The model under review builds one solid part; all positions refer to its coordinate system, in mm. A direction names the side the tool comes from. Round coordinates to 2 decimals unless told otherwise and drop trailing zeros. Write each loop counter-clockwise with the first axis right and the second up, starting at its lowest first coordinate (ties: lowest second). Pieces come first, ordered by that corner, then holes. Notation, with made-up numbers: (72.5, 55.5) -> (101.5, 55.5) arc R16 cw to (101.5, 74.5) -> close; hole circle Ø11 at (27, 71). An arc over 180 degrees is marked (long way). Answer as a JSON object with one key per item and string values. Group by question number.
1) Mouldability with a two-part tool opening along Y and no side actions: class faces 1 (the cylindrical face through (-3.955, 12.325, -5.158)), 2 (the flat face through (-8, 120, 0)), 3 (the flat face through (-8, 23, 0)), 4 (the cylindrical face through (-10.74, 59.51, -2.38)) as pulls with the +Y half, pulls with the -Y half, needs draft (parallel to the pull), parting line crosses it, or undercut.
2) We need section A-A, the plane x = 0. Write out the cut boundary in (y, z), then the cut area to 3 significant figures.
3) We need section D-D, the plane y = 69.5. Write out the cut boundary in (x, z).
4) We need section B-B, the plane z = 3.75. Write out the cut boundary in (x, y).
5) Insertion check: pin 1 Ø1.5 at (x, y) = (-6.5, 105.5) entering from -Z; pin 2 Ø6 at (x, z) = (0, 0.5) entering from +Y; pin 3 Ø10 at (y, z) = (40, -6.5) entering from +X; pin 4 Ø6 at (y, z) = (94.5, 5) entering from -X. Each pin has a flat end and moves straight along its axis. Give the tip position at first contact, or say it passes through.
6) We need section C-C, the plane y = 112. Write out the cut boundary in (x, z), then the cut area to 3 significant figures.
7) Machinability: for faces 5 (the cylindrical face through (0.33, 11.339, -7.493)), 6 (the flat face through (3, 0, -6)), 7 (the flat face through (3, 97, 8.2)), 8 (the flat face through (-5, 25, 5)), which of the approach directions +Z, -Z, +X, -X, +Y, -Y give a long, thin tool a straight path to every point of the face, cutting with its end or side? Answer none if there is none.
8) To check wall thickness, follow probe 1 along Y at (x, z) = (5.75, -9); probe 2 along X at (y, z) = (10.25, 0); probe 3 along X at (y, z) = (111, 0). State the ranges of each line that lie inside material, in increasing order. Write a range as [from, to].
from build123d import *

# Parameters (mm, degrees)
SKETCH1_R           = 7.5
SKETCH1_R_2         = 6.5
BOSS_EXTRUDE1_DEPTH = 23
SKETCH2_R           = 12.5
SKETCH2_R_2         = 6.5
BOSS_EXTRUDE2_DEPTH = 2
SKETCH3_R           = 12.5
SKETCH3_R_2         = 11
BOSS_EXTRUDE3_DEPTH = 70
SKETCH4_R           = 12.5
SKETCH4_R_2         = 7.5
BOSS_EXTRUDE4_DEPTH = 2
SKETCH5_R           = 8.5
SKETCH5_R_2         = 7.5
BOSS_EXTRUDE5_DEPTH = 23


with BuildPart() as part:
    # Sketch1 → Boss-Extrude1 (new body)
    with BuildSketch(Plane(origin=(0, 0, 0), x_dir=(1, 0, 0), z_dir=(0, 1, 0))):
        with Locations(Location((0, 0, 0), (0, 0, 270))):
            Circle(SKETCH1_R)
        with Locations(Location((0, 0, 0), (0, 0, 270))):
            Circle(SKETCH1_R_2, mode=Mode.SUBTRACT)
    extrude(amount=BOSS_EXTRUDE1_DEPTH)

    # Sketch2 → Boss-Extrude2 (add)
    with BuildSketch(Plane(origin=(0, 23, 0), x_dir=(1, 0, 0), z_dir=(0, 1, 0))):
        with Locations(Location((0, 0, 0), (0, 0, 270))):
            Circle(SKETCH2_R)
        with Locations(Location((0, 0, 0), (0, 0, 270))):
            Circle(SKETCH2_R_2, mode=Mode.SUBTRACT)
    extrude(amount=BOSS_EXTRUDE2_DEPTH)

    # Sketch3 → Boss-Extrude3 (add)
    with BuildSketch(Plane(origin=(0, 25, 0), x_dir=(1, 0, 0), z_dir=(0, 1, 0))):
        with Locations(Location((0, 0, 0), (0, 0, 270))):
            Circle(SKETCH3_R)
        with Locations(Location((0, 0, 0), (0, 0, 270))):
            Circle(SKETCH3_R_2, mode=Mode.SUBTRACT)
    extrude(amount=BOSS_EXTRUDE3_DEPTH)

    # Sketch4 → Boss-Extrude4 (add)
    with BuildSketch(Plane(origin=(0, 95, 0), x_dir=(1, 0, 0), z_dir=(0, 1, 0))):
        with Locations(Location((0, 0, 0), (0, 0, 270))):
            Circle(SKETCH4_R)
        with Locations(Location((0, 0, 0), (0, 0, 270))):
            Circle(SKETCH4_R_2, mode=Mode.SUBTRACT)
    extrude(amount=BOSS_EXTRUDE4_DEPTH)

    # Sketch5 → Boss-Extrude5 (add)
    with BuildSketch(Plane(origin=(0, 97, 0), x_dir=(1, 0, 0), z_dir=(0, 1, 0))):
        with Locations(Location((0, 0, 0), (0, 0, 270))):
            Circle(SKETCH5_R)
        with Locations(Location((0, 0, 0), (0, 0, 270))):
            Circle(SKETCH5_R_2, mode=Mode.SUBTRACT)
    extrude(amount=BOSS_EXTRUDE5_DEPTH)


solid = part.part
Here are the results:
{
 "1": {"face 1": "needs draft", "face 2": "pulls with the +Y half", "face 3": "pulls with the -Y half", "face 4": "undercut"},
 "2": {"outline": "(0, -7.5) -> (23, -7.5) -> (23, -12.5) -> (97, -12.5) -> (97, -8.5) -> (120, -8.5) -> (120, -7.5) -> (95, -7.5) -> (95, -11) -> (25, -11) -> (25, -6.5) -> (0, -6.5) -> close; (0, 6.5) -> (25, 6.5) -> (25, 11) -> (95, 11) -> (95, 7.5) -> (120, 7.5) -> (120, 8.5) -> (97, 8.5) -> (97, 12.5) -> (23, 12.5) -> (23, 7.5) -> (0, 7.5) -> close", "area": "346 mm^2"},
 "3": {"outline": "circle Ø25 at (0, 0); hole circle Ø22 at (0, 0)"},
 "4": {"outline": "(-11.92, 23) -> (-6.5, 23) -> (-6.5, 0) -> (-5.31, 0) -> (-5.31, 25) -> (-10.34, 25) -> (-10.34, 95) -> (-6.5, 95) -> (-6.5, 120) -> (-7.63, 120) -> (-7.63, 97) -> (-11.92, 97) -> close; (5.31, 0) -> (6.5, 0) -> (6.5, 23) -> (11.92, 23) -> (11.92, 97) -> (7.63, 97) -> (7.63, 120) -> (6.5, 120) -> (6.5, 95) -> (10.34, 95) -> (10.34, 25) -> (5.31, 25) -> close"},
 "5": {"pin 1": "stops at z = -6.26", "pin 2": "passes through", "pin 3": "stops at x = 12.41", "pin 4": "stops at x = -12.34"},
 "6": {"outline": "circle Ø17 at (0, 0); hole circle Ø15 at (0, 0)", "area": "50.3 mm^2"},
 "7": {"face 5": "-Y", "face 6": "+Z, -Z, +X, -X, -Y", "face 7": "+Y", "face 8": "none"},
 "8": {"probe 1": "y = [23, 25], [95, 97]", "probe 2": "x = [-7.5, -6.5], [6.5, 7.5]", "probe 3": "x = [-8.5, -7.5], [7.5, 8.5]"}
}
